The drawing under review shows one solid part. Ordinate dimensions are in mm from its lowest x, y, z. Coordinates: 2 decimals unless noted, no trailing zeros. Loops run counter-clockwise (first coordinate to the right, second up) from the corner with the lowest first, then second, coordinate; pieces in that order, holes last. Notation, with made-up numbers: (15.5, 29) -> (59.5, 29) arc R15 ccw to (59.5, 52) -> close; hole circle Ø7 at (-22, 0). An arc over 180 degrees is marked (long way). Use a Markdown table: item, result.
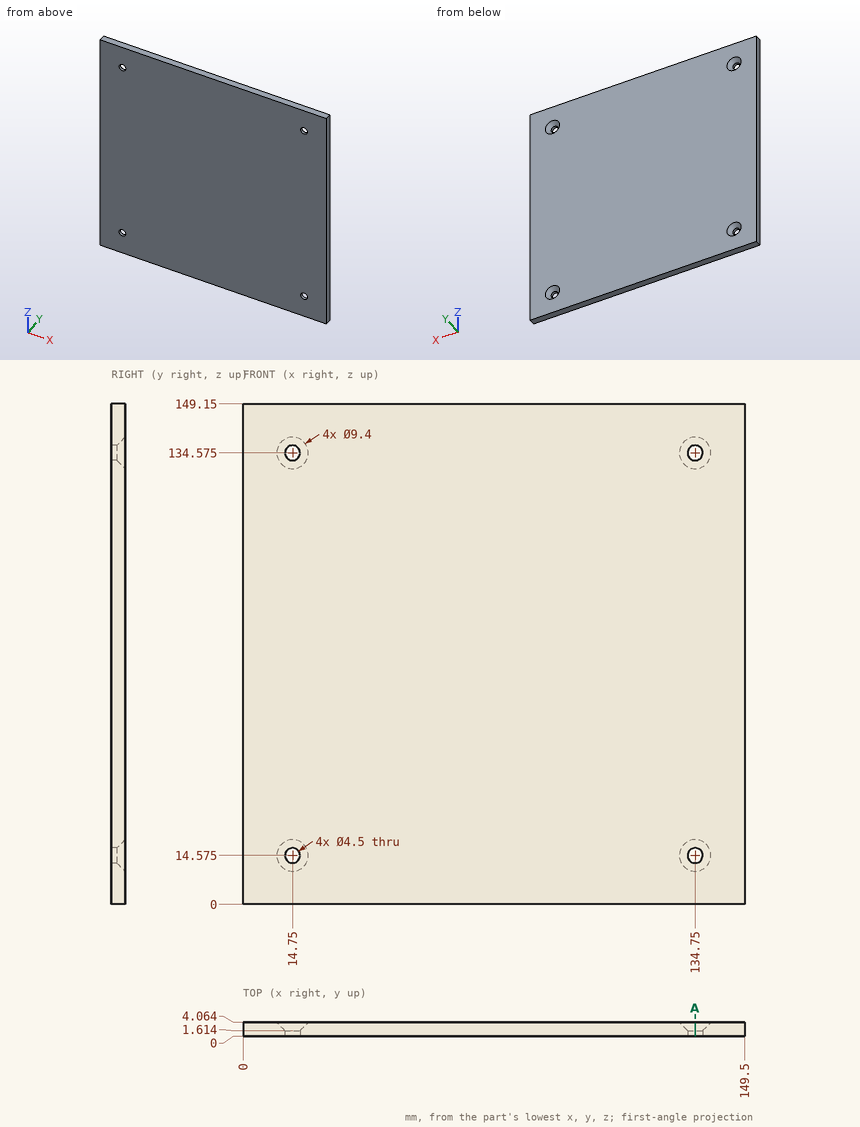
(1) Take a section at A-A on x = 134.75. Write out the cut boundary in (y, z) (3 decimals), plus the area to 3 significant figures.
Found:
| item | result |
|---|---|
| outline | (0, 0) -> (4.064, 0) -> (4.064, 9.875) -> (1.614, 12.325) -> (0, 12.325) -> close; (0, 16.825) -> (1.614, 16.825) -> (4.064, 19.275) -> (4.064, 129.875) -> (1.614, 132.325) -> (0, 132.325) -> close; (0, 136.825) -> (1.614, 136.825) -> (4.064, 139.275) -> (4.064, 149.15) -> (0, 149.15) -> close |
| area | 558 mm^2 |
(2) For line 1 along Z through (x, y) = (14.75, 0.4) (3 decimals); line 2 along X through (y, z) = (0.95, 14.5); line 3 along Z through (x, y) = (11, 3.95), list the stretches that pass through material, from the lowest coordinate up.
Found:
| item | result |
|---|---|
| line 1 | z = 0 to 12.325, 16.825 to 132.325, 136.825 to 149.15 |
| line 2 | x = 0 to 12.5, 17 to 132.5, 137 to 149.5 |
| line 3 | z = 0 to 11.94, 17.21 to 131.94, 137.21 to 149.15 |
(3) For pin 1 Ø4 at (x, z) = (134.75, 14.575) entering from -Y, flat-tipped, find the tip position at first contact; note if it passes through.
Found:
| item | result |
|---|---|
| pin 1 | passes through |
